Geometry: final body of the model. Coordinates: model frame, mm. Face numbers are marked on the shaded views. Give positions to 0.01 mm unless a question says otherwise; leave off trailing zeros. Order: outer loops, then holes, each group sorted by start corner. A loop starts at its lowest first (then second) coordinate and runs counter-clockwise, first axis right, second up. Notation, with made-up numbers: (-28.5, 52.5) -> (24.5, 52.5) arc R9 ccw to (24.5, 64.5) -> close; hole circle Ø10 at (75.5, -33.5). An arc over 180 degrees is marked (long way). One line per question, with ' | ' between items. Start each with the question number.
(1) Section A-A (y = 0). Return loops of the section in (x, z), then the cut area to 3 significant figures.
(2) Ray query, L1, parallel to Y at x = 0, z = 12.5; L2, parallel to X at y = -4, z = 18; L3, parallel to X at y = -2.25, z = 15.5. Return the intervals inside material, ascending.
(3) First-contact query: pin 1 Ø0.8 at (x, z) = (-7, -3.5) entering from +Y; pin 2 Ø0.5 at (x, y) = (-7, -2.5) entering from +Z; pin 3 Ø3 at (y, z) = (1, 28.5) entering from +X; pin 4 Ø5 at (y, z) = (1, 20.5) entering from +X. Flat tips, straight axial feed; report the tip coordinate or a pass-through.
(4) Section C-C (z = 29.5). Return loops of the section in (x, y), then the cut area to 3 significant figures.
(5) Mould query, pull axis X, two halves, no side actions, for the marked faces 1 and 2. Classes: +X half, -X half, draft (parallel to the pull), parting line (faces both ways), or undercut.
(6) Section D-D (z = 16). Return loops of the section in (x, y), then the cut area to 3 significant figures.
(7) Section B-B (x = -5). Return loops of the section in (y, z), then the cut area to 3 significant figures.
```python
from build123d import *

# Parameters (mm, degrees)
ESBO_O2_R                = 7.5
ESBO_O2_R_2              = 6.5
RESSALTO_EXTRUS_O1_DEPTH = 23.5
RESSALTO_EXTRUS_O2_DEPTH = 1


with BuildPart() as part:
    # Esboço2 → Ressalto-extrusão1 (new body)
    with BuildSketch(Plane.XY):
        Circle(ESBO_O2_R)
        Circle(ESBO_O2_R_2, mode=Mode.SUBTRACT)
    extrude(amount=RESSALTO_EXTRUS_O1_DEPTH)

    # Esboço3 → Ressalto-extrusão2 (add)
    with BuildSketch(Plane(origin=(-7.5, 0, 0), x_dir=(0, 0, -1), z_dir=(1, 0, 0))):
        with BuildLine():
            Line((5, 2), (0, 2))
            Line((0, 2), (0, 3))
            Line((0, 3), (5, 3))
            ThreePointArc((5, 3), (8, 0), (5, -3))
            Line((5, -3), (0, -3))
            Line((0, -3), (0, -2))
            Line((0, -2), (5, -2))
            ThreePointArc((5, -2), (7, 0), (5, 2))
        make_face()
        with BuildLine():
            Line((-28.5, 3), (-23.5, 3))
            Line((-23.5, 3), (-23.5, 2))
            Line((-23.5, 2), (-28.5, 2))
            ThreePointArc((-28.5, 2), (-30.5, 0), (-28.5, -2))
            Line((-28.5, -2), (-23.5, -2))
            Line((-23.5, -2), (-23.5, -3))
            Line((-23.5, -3), (-28.5, -3))
            ThreePointArc((-28.5, -3), (-31.5, 0), (-28.5, 3))
        make_face()
    extrude(amount=RESSALTO_EXTRUS_O2_DEPTH)


solid = part.part
```
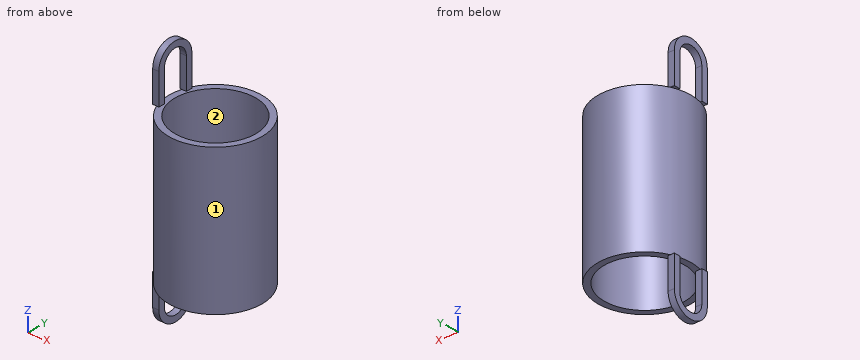
Response:
1) outline: (-7.5, -8) -> (-6.5, -8) -> (-6.5, -7) -> (-7.5, -7) -> close; (-7.5, 0) -> (-6.5, 0) -> (-6.5, 23.5) -> (-7.5, 23.5) -> close; (-7.5, 30.5) -> (-6.5, 30.5) -> (-6.5, 31.5) -> (-7.5, 31.5) -> close; (6.5, 0) -> (7.5, 0) -> (7.5, 23.5) -> (6.5, 23.5) -> close | area: 49.0 mm^2
2) L1: y = -7.5 to -6.5, 6.5 to 7.5 | L2: x = -6.34 to -5.12, 5.12 to 6.34 | L3: x = -7.15 to -6.1, 6.1 to 7.15
3) pin 1: stops at y = 3 | pin 2: stops at z = 30.48 | pin 3: stops at x = -6.5 | pin 4: stops at x = 7.5
4) outline: (-7.5, -2.83) -> (-6.5, -2.83) -> (-6.5, -1.73) -> (-7.5, -1.73) -> close; (-7.5, 1.73) -> (-6.5, 1.73) -> (-6.5, 2.83) -> (-7.5, 2.83) -> close | area: 2.19 mm^2
5) face 1: parting line | face 2: undercut
6) outline: circle Ø15 at (0, 0); hole circle Ø13 at (0, 0) | area: 44.0 mm^2
7) outline: (-5.59, 0) -> (-4.15, 0) -> (-4.15, 23.5) -> (-5.59, 23.5) -> close; (4.15, 0) -> (5.59, 0) -> (5.59, 23.5) -> (4.15, 23.5) -> close | area: 67.5 mm^2
